```python
from build123d import *

# Parameters (mm, degrees)
CROQUIS1_W              = 80
CROQUIS1_H              = 60
CROQUIS1_R              = 1.5
CROQUIS1_W_2            = 6
CROQUIS1_H_2            = 25
CROQUIS1_W_3            = 10
CROQUIS1_H_3            = 20
CROQUIS1_H_4            = 10
CROQUIS1_W_4            = 5
CROQUIS1_H_5            = 6.5
SALIENTE_EXTRUIR1_DEPTH = 15
CORTAR_EXTRUIR1_DEPTH   = 10
CROQUIS3_R              = 1.5
CORTAR_EXTRUIR2_DEPTH   = 25
CORTAR_EXTRUIR3_START   = -25
CROQUIS6_R              = 1.5
CORTAR_EXTRUIR3_DEPTH   = 25
CROQUIS8_W              = 16
CROQUIS8_H              = 17.848141148
CROQUIS8_R              = 1.5
SALIENTE_EXTRUIR2_DEPTH = 5
CORTAR_EXTRUIR4_START   = -55
CORTAR_EXTRUIR4_DEPTH   = 8
CROQUIS10_R             = 1.5
CROQUIS10_W             = 6
CROQUIS10_H             = 12
CORTAR_EXTRUIR5_DEPTH   = 16
CORTAR_EXTRUIR6_DEPTH   = 10


with BuildPart() as part:
    # Croquis1 → Saliente-Extruir1 (new body)
    # profile 1 of 13: a face of its own
    with BuildSketch(Plane(origin=(0, 0, 0), x_dir=(1, 0, 0), z_dir=(0, 1, 0))):
        with Locations((0, -10)):
            Rectangle(CROQUIS1_W, CROQUIS1_H)
        with Locations(Location((18, -16.5, 0), (0, 0, 270))):
            Circle(CROQUIS1_R, mode=Mode.SUBTRACT)
        with Locations(Location((-11, -16.5, 0), (0, 0, 270))):
            Circle(CROQUIS1_R, mode=Mode.SUBTRACT)
        with Locations(Location((18, 16.5, 0), (0, 0, 270))):
            Circle(CROQUIS1_R, mode=Mode.SUBTRACT)
        with Locations(Location((-11, 16.5, 0), (0, 0, 270))):
            Circle(CROQUIS1_R, mode=Mode.SUBTRACT)
        with Locations((18, 0)):
            Rectangle(CROQUIS1_W_2, CROQUIS1_H_2, mode=Mode.SUBTRACT)
        Polygon((6.711696879, 3.875), (0, 7.75), (-6.711696879, 3.875), (-6.711696879, -3.875), (0, -7.75), (6.711696879, -3.875), align=None, mode=Mode.SUBTRACT)
        with Locations((-11, 0)):
            Rectangle(CROQUIS1_W_2, CROQUIS1_H_2, mode=Mode.SUBTRACT)
    # profile 2 of 13: a face of its own
    with BuildSketch(Plane(origin=(0, 0, 0), x_dir=(1, 0, 0), z_dir=(0, 1, 0))):
        with Locations((-45, -10)):
            Rectangle(CROQUIS1_W_3, CROQUIS1_H_3)
    # profile 3 of 13: a face of its own
    with BuildSketch(Plane(origin=(0, 0, 0), x_dir=(1, 0, 0), z_dir=(0, 1, 0))):
        with Locations((-45, -35)):
            Rectangle(CROQUIS1_W_3, CROQUIS1_H_4)
    # profile 4 of 13: a face of its own
    with BuildSketch(Plane(origin=(0, 0, 0), x_dir=(1, 0, 0), z_dir=(0, 1, 0))):
        with Locations((-52.5, -10)):
            Rectangle(CROQUIS1_W_4, CROQUIS1_H)
    # profile 5 of 13: a face of its own
    with BuildSketch(Plane(origin=(0, 0, 0), x_dir=(1, 0, 0), z_dir=(0, 1, 0))):
        with Locations((-45, 15)):
            Rectangle(CROQUIS1_W_3, CROQUIS1_H_4)
    # profile 6 of 13: a face of its own
    with BuildSketch(Plane(origin=(0, 0, 0), x_dir=(1, 0, 0), z_dir=(0, 1, 0))):
        with Locations((45, 15)):
            Rectangle(CROQUIS1_W_3, CROQUIS1_H_4)
    # profile 7 of 13: a face of its own
    with BuildSketch(Plane(origin=(0, 0, 0), x_dir=(1, 0, 0), z_dir=(0, 1, 0))):
        with Locations((52.5, -10)):
            Rectangle(CROQUIS1_W_4, CROQUIS1_H)
    # profile 8 of 13: a face of its own
    with BuildSketch(Plane(origin=(0, 0, 0), x_dir=(1, 0, 0), z_dir=(0, 1, 0))):
        with Locations((45, -10)):
            Rectangle(CROQUIS1_W_3, CROQUIS1_H_3)
    # profile 9 of 13: a face of its own
    with BuildSketch(Plane(origin=(0, 0, 0), x_dir=(1, 0, 0), z_dir=(0, 1, 0))):
        with Locations((45, -35)):
            Rectangle(CROQUIS1_W_3, CROQUIS1_H_4)
    # profile 10 of 13: a face of its own
    with BuildSketch(Plane(origin=(0, 0, 0), x_dir=(1, 0, 0), z_dir=(0, 1, 0))):
        with Locations((-11, 9.25)):
            Rectangle(CROQUIS1_W_2, CROQUIS1_H_5)
    # profile 11 of 13: a face of its own
    with BuildSketch(Plane(origin=(0, 0, 0), x_dir=(1, 0, 0), z_dir=(0, 1, 0))):
        with Locations((-11, -9.25)):
            Rectangle(CROQUIS1_W_2, CROQUIS1_H_5)
    # profile 12 of 13: a face of its own
    with BuildSketch(Plane(origin=(0, 0, 0), x_dir=(1, 0, 0), z_dir=(0, 1, 0))):
        with Locations((18, 9.25)):
            Rectangle(CROQUIS1_W_2, CROQUIS1_H_5)
    # profile 13 of 13: a face of its own
    with BuildSketch(Plane(origin=(0, 0, 0), x_dir=(1, 0, 0), z_dir=(0, 1, 0))):
        with Locations((18, -9.25)):
            Rectangle(CROQUIS1_W_2, CROQUIS1_H_5)
    extrude(amount=SALIENTE_EXTRUIR1_DEPTH)

    # Croquis2 → Cortar-Extruir1 (cut)
    with BuildSketch(Plane.XZ):
        Polygon((-7.391560818, 16.5), (-9.195780409, 19.625), (-12.804219591, 19.625), (-14.608439182, 16.5), (-12.804219591, 13.375), (-9.195780409, 13.375), align=None)
        Polygon((21.608439182, 16.5), (19.804219591, 19.625), (16.195780409, 19.625), (14.391560818, 16.5), (16.195780409, 13.375), (19.804219591, 13.375), align=None)
        Polygon((-7.391560818, -16.5), (-9.195780409, -13.375), (-12.804219591, -13.375), (-14.608439182, -16.5), (-12.804219591, -19.625), (-9.195780409, -19.625), align=None)
        Polygon((21.608439182, -16.5), (19.804219591, -13.375), (16.195780409, -13.375), (14.391560818, -16.5), (16.195780409, -19.625), (19.804219591, -19.625), align=None)
    extrude(amount=-CORTAR_EXTRUIR1_DEPTH, mode=Mode.SUBTRACT)

    # Croquis3 → Cortar-Extruir2 (cut)
    with BuildSketch(Plane(origin=(55, 0, 0), x_dir=(0, 0, -1), z_dir=(1, 0, 0))):
        with Locations((-25, 7.5)):
            Circle(CROQUIS3_R)
        with Locations((5, 7.5)):
            Circle(CROQUIS3_R)
    extrude(amount=-CORTAR_EXTRUIR2_DEPTH, mode=Mode.SUBTRACT)

    # Croquis6 → Cortar-Extruir3 (cut)
    with BuildSketch(Plane.ZY.offset(55).offset(CORTAR_EXTRUIR3_START)):
        with Locations(Location((-5, 7.5, 0), (0, 0, 180))):
            Circle(CROQUIS6_R)
        with Locations(Location((25, 7.5, 0), (0, 0, 180))):
            Circle(CROQUIS6_R)
    extrude(amount=CORTAR_EXTRUIR3_DEPTH, mode=Mode.SUBTRACT)

    # Croquis8 → Saliente-Extruir2 (add)
    with BuildSketch(Plane(origin=(0, 15, 0), x_dir=(1, 0, 0), z_dir=(0, 1, 0))):
        Rectangle(CROQUIS8_W, CROQUIS8_H)
        with Locations(Location((0, 0, 0), (0, 0, 270))):
            Circle(CROQUIS8_R, mode=Mode.SUBTRACT)
    extrude(amount=-SALIENTE_EXTRUIR2_DEPTH)

    # Croquis9 → Cortar-Extruir4 (cut, symmetric)
    with BuildSketch(Plane(origin=(55, 0, 0), x_dir=(0, 0, -1), z_dir=(1, 0, 0)).offset(CORTAR_EXTRUIR4_START)):
        Polygon((-40, 3), (-12.5, 15), (-40, 15), align=None)
    extrude(amount=CORTAR_EXTRUIR4_DEPTH, both=True, mode=Mode.SUBTRACT)

    # Croquis10 → Cortar-Extruir5 (cut)
    with BuildSketch(Plane(origin=(0, 15, 0), x_dir=(1, 0, 0), z_dir=(0, 1, 0))):
        with Locations(Location((25, -0.5, 0), (0, 0, 270))):
            Circle(CROQUIS10_R)
        with Locations(Location((25, -24.5, 0), (0, 0, 270))):
            Circle(CROQUIS10_R)
        with Locations((25, -12.5)):
            Rectangle(CROQUIS10_W, CROQUIS10_H)
    extrude(amount=-CORTAR_EXTRUIR5_DEPTH, mode=Mode.SUBTRACT)

    # Croquis11 → Cortar-Extruir6 (cut)
    with BuildSketch(Plane.XZ):
        Polygon((28.608439182, 24.5), (26.804219591, 27.625), (23.195780409, 27.625), (21.391560818, 24.5), (23.195780409, 21.375), (26.804219591, 21.375), align=None)
        Polygon((28.608439182, 0.5), (26.804219591, 3.625), (23.195780409, 3.625), (21.391560818, 0.5), (23.195780409, -2.625), (26.804219591, -2.625), align=None)
    extrude(amount=-CORTAR_EXTRUIR6_DEPTH, mode=Mode.SUBTRACT)


solid = part.part
```
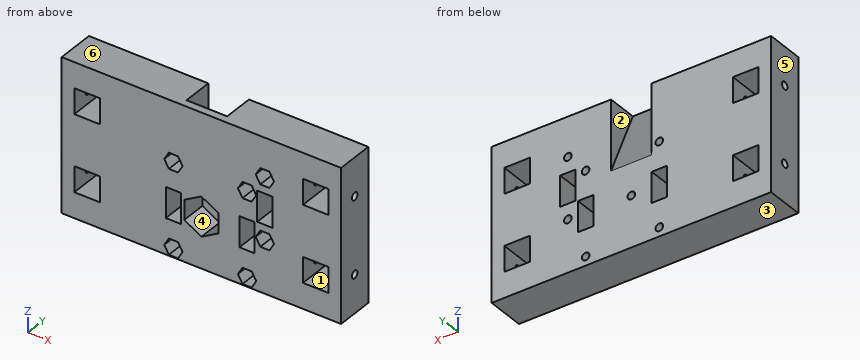
For this review, take the finished solid that the model builds, in its own axes (mm). Face numbers are marked on the shaded views. A direction names the side the tool comes from. Coordinates: 2 decimals unless noted, no trailing zeros. Order: outer loops, then holes, each group sorted by start corner. A loop starts at its lowest first (then second) coordinate and runs counter-clockwise, first axis right, second up. Notation, with made-up numbers: (9.25, -24) -> (37.25, -24) arc R20 cw to (37.25, -3) -> close; hole circle Ø11 at (-9, 83.5). An arc over 180 degrees is marked (long way). Use CSV: the item, a comma, the result in double quotes. Start each with the question number.
Item 1: For the marked faces 1, 2 and 3, list the 3-axis set-ups (+Z, -Z, +X, -X, +Y, -Y) from which the entire face can be reached by the end or side of a thin tool; tool diameter is ignored.
Item 2: Wall thickness on probe 1 along Z at (x, y) = (-52.95, 7.5); probe 2 along X at (y, z) = (11.15, 24.5); probe 3 along Z at (x, y) = (18, 11.1): over which ranges is each line inside the solid? List them lowest first.
Item 3: Insertion check: pin 1 (2.5 mm diameter, centred on y = 7.5, z = 25, fed in from +X); pin 2 (3 mm diameter, centred on x = 24.5, z = 2, fed in from -Y); pin 3 (1.5 mm diameter, centred on y = 8, z = 24.5, fed in from -X). Each pin has a flat end and moves straight along its axis. Give the tip position at first contact, or say it passes through.
Item 4: Draft analysis for pull direction X (two halves, no side actions). For the marked faces 4, 5 and 6, state which applies: pulls with the +X half, pulls with the -X half, needs draft (parallel to the pull), parting line crosses it, or undercut.
Item 5: We need section A-A, the plane x = -47. Give the boundary of the cut face in (y, z), then the cut area to 3 significant figures.
Item 6: We need section B-B, the plane y = 11.75. Give the number of separate pieces and of enclosed holes in the cut face, then the cut area to 3 significant figures.
Derived:
1,face 1,"+Y, -Y"
1,face 2,"+Z, +Y"
1,face 3,"-Z, +X, -X, +Y, -Y"
2,probe 1,"z = -20 to -6.5, -3.5 to 23.5, 26.5 to 40"
2,probe 2,"x = -55 to -50, -40 to -8, 8 to 23.5, 26.5 to 40, 50 to 55"
2,probe 3,"z = -20 to -18, -15 to -6, 6 to 15, 18 to 40"
3,pin 1,"stops at x = 30"
3,pin 2,"stops at y = 10"
3,pin 3,"stops at x = -30"
4,face 4,"undercut"
4,face 5,"pulls with the -X half"
4,face 6,"needs draft"
5,outline,"(0, -20) -> (15, -20) -> (15, -10) -> (0, -10) -> close; (0, 0) -> (15, 0) -> (15, 20) -> (0, 20) -> close; (0, 30) -> (15, 30) -> (15, 40) -> (0, 40) -> close"
5,area,"600 mm^2"
6,separate pieces,"1"
6,enclosed holes,"14"
6,area,"5,610 mm^2"
